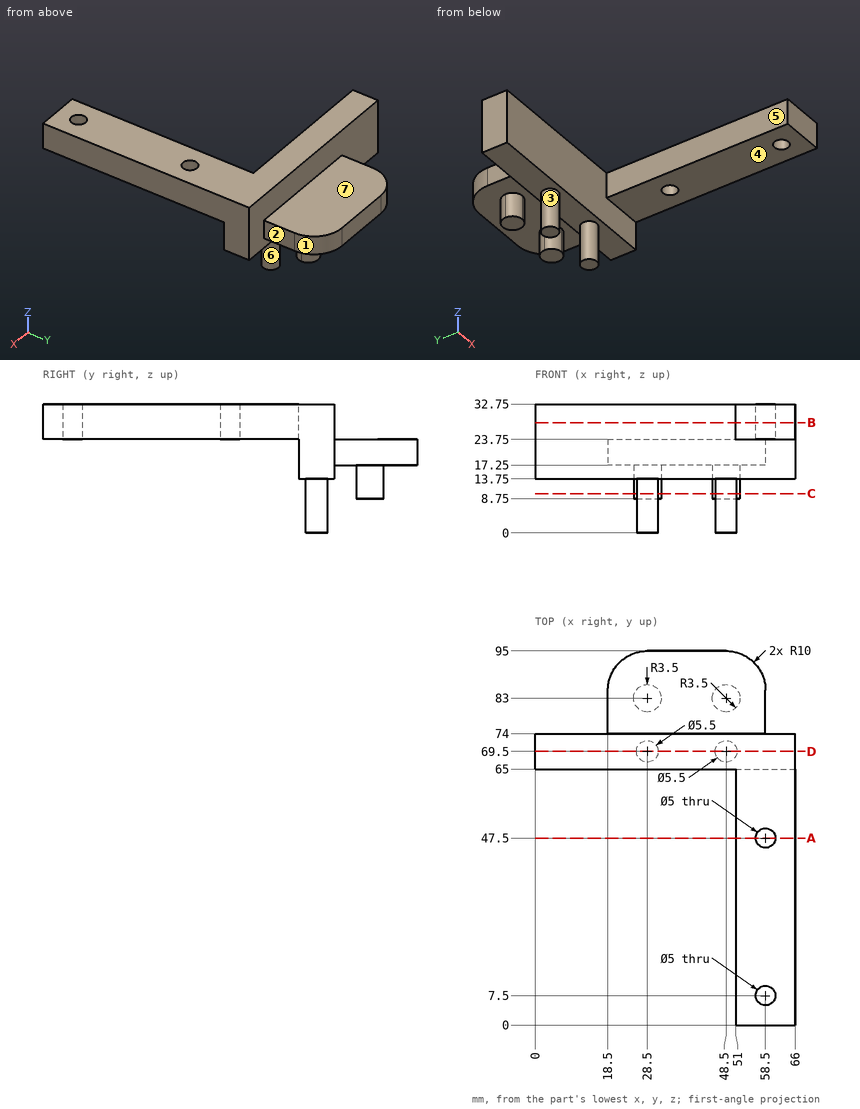
Drawing for the job (mm, zero at the part's lowest x, y, z). A direction names the side the tool comes from. Round coordinates to 2 decimals unless told otherwise and drop trailing zeros. Loops run counter-clockwise (first coordinate to the right, second up) from the corner with the lowest first, then second, coordinate; pieces in that order, holes last.
1. Wall check: probe 1 along Y at (x, z) = (58.5, 26.5); probe 2 along Y at (x, z) = (29, 25.5); probe 3 along X at (y, z) = (40.5, 24). Give the ranges that are in metal, low to high.
Check values:
probe 1: y = 0 to 5, 10 to 45, 50 to 74
probe 2: y = 65 to 74
probe 3: x = 51 to 66
2. Band-saw the part on C-C, the plane z = 10. List the corners of the cut face in (x, y), and give its area (3 significant figures).
Check values:
outline: circle Ø7 at (28.5, 83); circle Ø5.5 at (28.5, 69.5); circle Ø7 at (48.5, 83); circle Ø5.5 at (48.5, 69.5)
area: 124 mm2
3. Band-saw the part on D-D, the plane y = 69.5. List the corners of the cut face in (x, z), and give its area (3 significant figures).
Check values:
outline: (0, 13.75) - (25.75, 13.75) - (25.75, 0) - (31.25, 0) - (31.25, 13.75) - (45.75, 13.75) - (45.75, 0) - (51.25, 0) - (51.25, 13.75) - (66, 13.75) - (66, 32.75) - (0, 32.75) - close
area: 1,410 mm2
4. Tool access for the marked faces 4, 5, 6 and 7: list every direction of +Z, -Z, +X, -X, +Y, -Y with a clear straight run to the whole face (end or side of a thin tool).
Check values:
face 4: -Z, +X, -X, -Y
face 5: +Z, -Z, -X, -Y
face 6: -Z
face 7: +Z, +X, -X, +Y
5. Drop flat-ended pins along their axis: P1, Ø10.5, axis at x = 46.5, y = 79.5, coming from the -Z side; P2, Ø4, axis at x = 56.5, z = 17, coming from the +Y side; P3, Ø10, axis at y = 34.5, z = 22, coming from the -X side; P4, Ø2, axis at y = 12, z = 21.5, coming from the +X side. Give the stop position or say it passes through.
Check values:
P1: stops at z = 8.75
P2: stops at y = 92.99
P3: stops at x = 51
P4: passes through
6. Band-saw the part on B-B, the plane z = 28. List the corners of the cut face in (x, y).
Check values:
outline: (0, 65) - (51, 65) - (51, 0) - (66, 0) - (66, 74) - (0, 74) - close; hole circle Ø5 at (58.5, 7.5); hole circle Ø5 at (58.5, 47.5)
7. Band-saw the part on A-A, the plane y = 47.5. List the corners of the cut face in (x, z), and give its area (3 significant figures).
Check values:
outline: (51, 23.75) - (56, 23.75) - (56, 32.75) - (51, 32.75) - close; (61, 23.75) - (66, 23.75) - (66, 32.75) - (61, 32.75) - close
area: 90.0 mm2
8. Mould opens along Y. For the marked faces 1, 2 and 3 say: +Y half, -Y half, draft (parallel to the pull), parting line (faces both ways), or undercut.
Check values:
face 1: +Y half
face 2: draft
face 3: undercut
